For this review, use the dimensioned drawing (mm, ordinates from the lowest corner) and the shaded views. Round coordinates to 2 decimals unless told otherwise and drop trailing zeros. Loops run counter-clockwise (first coordinate to the right, second up) from the corner with the lowest first, then second, coordinate; pieces in that order, holes last. Notation, with made-up numbers: (81, 85) - (104, 85) arc R24 cw to (104, 107) - close; hole circle Ø10 at (-24.75, 47.25). An arc over 180 degrees is marked (long way). Answer as CSV lines item,"result". Start each with the question number.
(1) Wall thickness on L1, parallel to Z at x = 3.2, y = 3.75; L2, parallel to Z at x = 4.25, y = 4; L3, parallel to Z at x = 5.75, y = 5: over which ranges is each line inside the solid? List them lowest first.
(2) For P1, Ø1.5, axis at x = 5.5, y = 3, coming from the +Z side, flat-tipped, find the tip position at first contact; note if it passes through.
(3) Consider section B-B (z = 14.75). Give the boundary of the cut face in (x, y).
(4) Mouldability with a two-part tool opening along X and no side actions: class the marked faces 1, 2, 3 and 4 as released by +X, released by -X, zero draft, split by the parting line, or undercut.
(5) Consider section C-C (y = 3.25). Give the boundary of the cut face in (x, z).
(6) Consider section A-A (x = 3.2). Give the boundary of the cut face in (y, z).
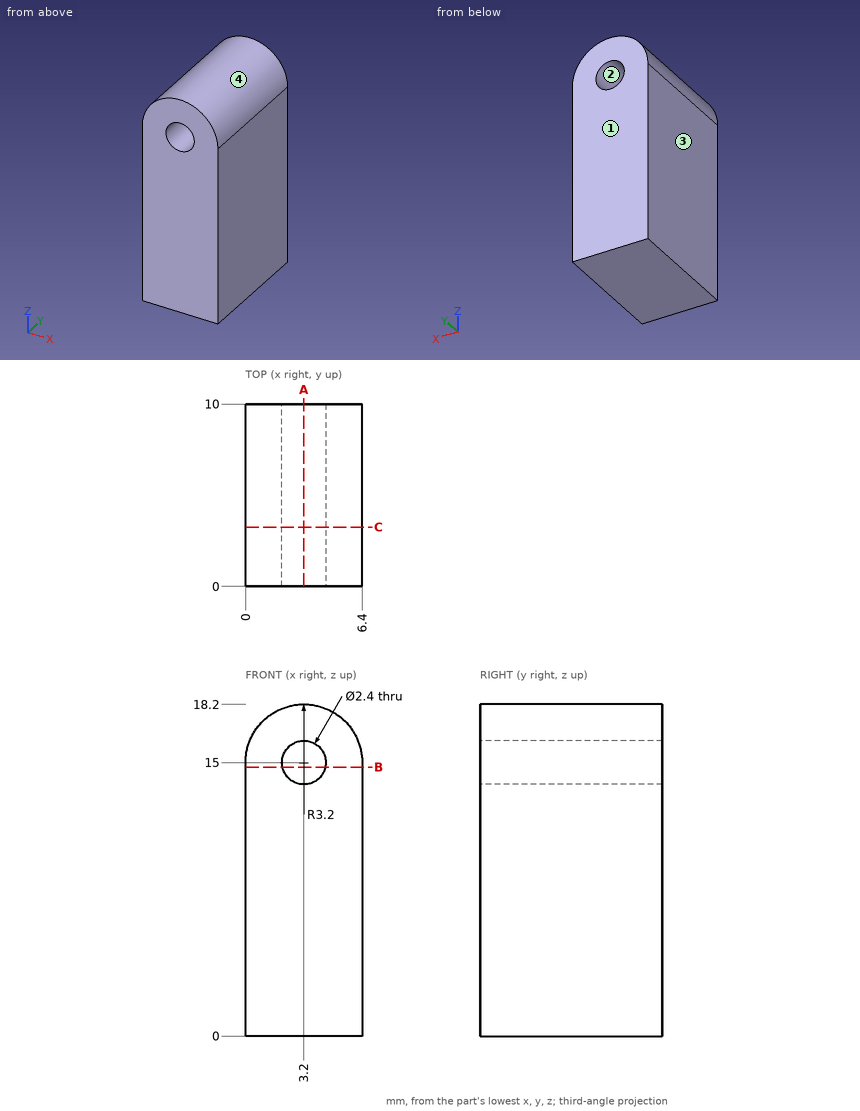
Determined:
1,L1,"z = 0 to 13.8, 16.2 to 18.2"
1,L2,"z = 0 to 14.42, 15.58 to 18.02"
1,L3,"z = 0 to 16.93"
2,P1,"stops at z = 17.8"
3,outline,"(0, 0) - (2.03, 0) - (2.03, 10) - (0, 10) - close; (4.37, 0) - (6.4, 0) - (6.4, 10) - (4.37, 10) - close"
4,face 1,"zero draft"
4,face 2,"undercut"
4,face 3,"released by -X"
4,face 4,"split by the parting line"
5,outline,"(0, 0) - (6.4, 0) - (6.4, 15) arc R3.2 ccw to (0, 15) - close; hole circle Ø2.4 at (3.2, 15)"
6,outline,"(0, 0) - (10, 0) - (10, 13.8) - (0, 13.8) - close; (0, 16.2) - (10, 16.2) - (10, 18.2) - (0, 18.2) - close"
